```python
from build123d import *

# Parameters (mm, degrees)
ESQUISSE1_R        = 2
BOSS_EXTRU_1_DEPTH = 3
CONG_1_R           = 4


with BuildPart() as part:
    # Esquisse1 → Boss.-Extru.1 (new body)
    with BuildSketch(Plane.XY):
        with BuildLine():
            Line((-5, -9.5), (9.5, -9.5))
            Line((9.5, -9.5), (9.5, 5))
            ThreePointArc((9.5, 5), (6.722075446, 9.157457896), (1.818019485, 8.181980515))
            Line((1.818019485, 8.181980515), (-8.181980515, -1.818019485))
            ThreePointArc((-8.181980515, -1.818019485), (-9.157457896, -6.722075446), (-5, -9.5))
        make_face()
        with Locations((5, 5)):
            Circle(ESQUISSE1_R, mode=Mode.SUBTRACT)
        with Locations((-5, -5)):
            Circle(ESQUISSE1_R, mode=Mode.SUBTRACT)
    extrude(amount=BOSS_EXTRU_1_DEPTH)

    # Congé1
    cong_1_edges = [part.edges().sort_by_distance(p)[0] for p in [
        (9.5, -9.5, 1.5),
    ]]
    fillet(cong_1_edges, radius=CONG_1_R)


solid = part.part
```
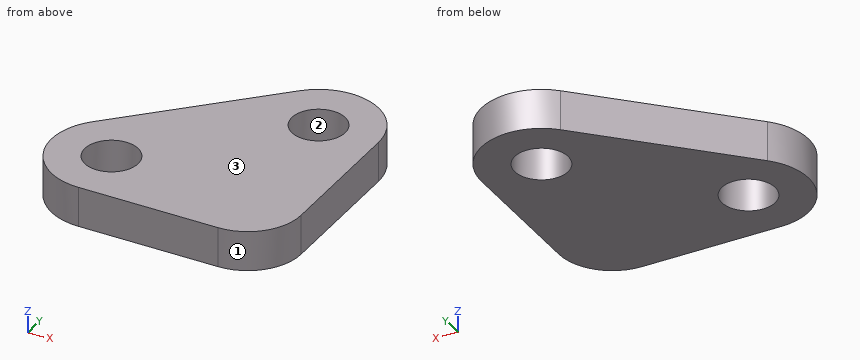
Check sheet for the modelled part. Datum: model origin and axes. Units: mm. Face numbers are marked on the shaded views. Coordinates: 2 decimals unless noted, no trailing zeros. Order: outer loops, then holes, each group sorted by start corner. A loop starts at its lowest first (then second) coordinate and runs counter-clockwise, first axis right, second up. Notation, with made-up numbers: M -16.5,-35 L 32.5,-35 A30 ccw 32.5,-1 Z; hole C 21.25,54 d4. An arc over 180 degrees is marked long. One line per question, with ' | ' between items. Start each with the question number.
Item 1: Sectioned sample at D-D on y = 0.75. Record the cut outline in (x, z), and give its area (3 significant figures).
Item 2: Sectioned sample at A-A on x = 5. Record the cut outline in (y, z), and give its area (3 significant figures).
Item 3: Sectioned sample at C-C on z = 0.9. Record the cut outline in (x, y), and give its area (3 significant figures).
Item 4: Mould release check, pull along X, two halves, no side actions. Record for the marked faces 1, 2 and 3: pulls with the +X half, pulls with the -X half, needs draft (parallel to the pull), parting line crosses it, or undercut.
Item 5: Sectioned sample at B-B on y = -5. Record the cut outline in (x, z), and give its area (3 significant figures).
Item 6: Material ranges on line 1 (Y direction, x = 5, z = 2.05); line 2 (X direction, y = -6.75, z = 2.6); line 3 (Y direction, x = -3.5, z = 0.75), recorded low to high.
Item 7: Gauge pin test, flat ends, axial feed: P1, Ø1.5, axis at y = 7.5, z = 0.5, coming from the +X side; P2, Ø1.5, axis at y = 1, z = 2, coming from the -X side. Record the tip position at first contact, or that the pin passes through.
Answer below:
1) outline: M -5.61,0 L 9.5,0 L 9.5,3 L -5.61,3 Z | area: 45.3 mm^2
2) outline: M -9.5,0 L 3,0 L 3,3 L -9.5,3 Z; M 7,0 L 9.5,0 L 9.5,3 L 7,3 Z | area: 45.0 mm^2
3) outline: M -8.18,-1.82 A4.5 ccw -5,-9.5 L 5.5,-9.5 A4 ccw 9.5,-5.5 L 9.5,5 A4.5 ccw 1.82,8.18 Z; hole C -5,-5 d4; hole C 5,5 d4 | area: 243 mm^2
4) face 1: pulls with the +X half | face 2: undercut | face 3: needs draft
5) outline: M -9.5,0 L -7,0 L -7,3 L -9.5,3 Z; M -3,0 L 9.5,0 L 9.5,3 L -3,3 Z | area: 45.0 mm^2
6) line 1: y = -9.5 to 3, 7 to 9.5 | line 2: x = -9.15 to -5.97, -4.03 to 9.3 | line 3: y = -9.5 to -6.32, -3.68 to 2.86
7) P1: stops at x = 9.15 | P2: stops at x = -6.11
